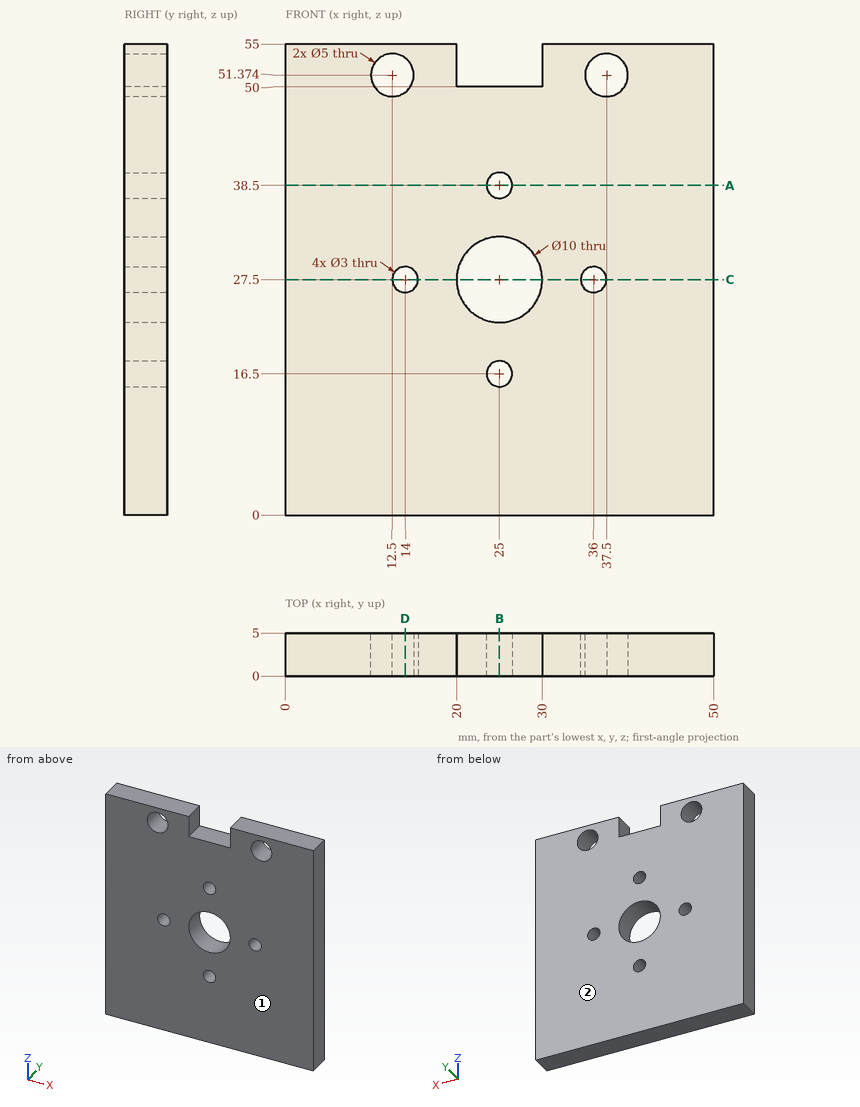
Input: dimensioned drawing with shaded views. Units: mm. Origin: part minimum x, y, z. Round coordinates to 2 decimals unless told otherwise and drop trailing zeros. Loops run counter-clockwise (first coordinate to the right, second up) from the corner with the lowest first, then second, coordinate; pieces in that order, holes last. Notation, with made-up numbers: (66.5, 77.25) -> (90.5, 77.25) arc R18 ccw to (90.5, 103.25) -> close; hole circle Ø7 at (88.25, 18.25). An arc over 180 degrees is marked (long way). One line per item, written item: value.
(1) Section D-D (x = 14). Return the cut outline in (y, z), plus the area to 3 significant figures.
Geometry check:
outline: (0, 0) -> (5, 0) -> (5, 26) -> (0, 26) -> close; (0, 29) -> (5, 29) -> (5, 49.37) -> (0, 49.37) -> close; (0, 53.37) -> (5, 53.37) -> (5, 55) -> (0, 55) -> close
area: 240 mm2
(2) Section A-A (z = 38.5). Return the cut outline in (x, y), plus the area to 3 significant figures.
Geometry check:
outline: (0, 0) -> (23.5, 0) -> (23.5, 5) -> (0, 5) -> close; (26.5, 0) -> (50, 0) -> (50, 5) -> (26.5, 5) -> close
area: 235 mm2
(3) Pin query (flat end, axial travel): pin 1 (1.5 mm diameter, centred on x = 24, y = 3, fed in from +Z). Return the tip coordinate at first contact, or that it passes through.
Geometry check:
pin 1: z = 50
(4) Material intervals for line 1 (Z direction, x = 25, y = 1.7); line 2 (Z direction, x = 13, y = 3.35); line 3 (Z direction, x = 36, y = 2.5), sorted ascending. Write a range as [from, to].
Geometry check:
line 1: [0, 15], [18, 22.5], [32.5, 37], [40, 50]
line 2: [0, 26.38], [28.62, 48.92], [53.82, 55]
line 3: [0, 26], [29, 49.37], [53.37, 55]
(5) Mould query, pull axis Y, two halves, no side actions, for the marked faces 1 and 2. Classes: pulls with the +Y half, pulls with the -Y half, needs draft (parallel to the pull), parting line crosses it, or undercut.
Geometry check:
face 1: pulls with the -Y half
face 2: pulls with the +Y half
(6) Section C-C (z = 27.5). Return the cut outline in (x, y).
Geometry check:
outline: (0, 0) -> (12.5, 0) -> (12.5, 5) -> (0, 5) -> close; (15.5, 0) -> (20, 0) -> (20, 5) -> (15.5, 5) -> close; (30, 0) -> (34.5, 0) -> (34.5, 5) -> (30, 5) -> close; (37.5, 0) -> (50, 0) -> (50, 5) -> (37.5, 5) -> close
(7) Section B-B (x = 25). Return the cut outline in (y, z).
Geometry check:
outline: (0, 0) -> (5, 0) -> (5, 15) -> (0, 15) -> close; (0, 18) -> (5, 18) -> (5, 22.5) -> (0, 22.5) -> close; (0, 32.5) -> (5, 32.5) -> (5, 37) -> (0, 37) -> close; (0, 40) -> (5, 40) -> (5, 50) -> (0, 50) -> close
